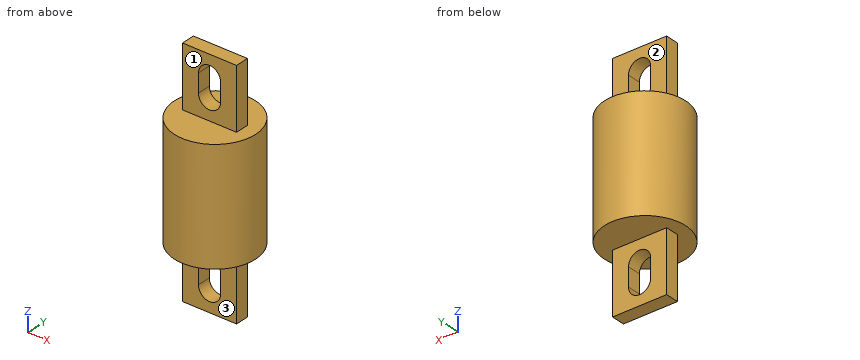
```python
from build123d import *

# Parameters (mm, degrees)
SKETCH1_R       = 19.05
FUSE_DEPTH      = 26.67
FUSE_DEPTH_BACK = 26.67
SKETCH2_W       = 25.4
SKETCH2_H       = 28.575
TAB_DEPTH       = 3.175


with BuildPart() as part:
    # Sketch1 → Fuse (new body, two sides)
    with BuildSketch(Plane.XY) as fuse_sk:
        Circle(SKETCH1_R)
    extrude(amount=FUSE_DEPTH)
    extrude(fuse_sk.sketch, amount=-FUSE_DEPTH_BACK)

    # Sketch2 → Tab (add, symmetric)
    with BuildSketch(Plane(origin=(0, 0, 0), x_dir=(1, 0, 0), z_dir=(0, 1, 0))):
        with Locations((0, 40.9575)):
            Rectangle(SKETCH2_W, SKETCH2_H)
        with BuildLine():
            Line((-5.207, 36.6395), (-5.207, 45.2755))
            ThreePointArc((-5.207, 45.2755), (0, 50.4825), (5.207, 45.2755))
            Line((5.207, 45.2755), (5.207, 36.6395))
            ThreePointArc((5.207, 36.6395), (0, 31.4325), (-5.207, 36.6395))
        make_face(mode=Mode.SUBTRACT)
    tab = extrude(amount=TAB_DEPTH, both=True)

    # Tab Mirror: Tab across plane
    add(tab.mirror(Plane.XY))


solid = part.part
```
Work out the finished part from the listing and answer in its coordinate system (mm). Face numbers are marked on the shaded views. A direction names the side the tool comes from. Give positions to 0.01 mm unless a question says otherwise; leave off trailing zeros. Order: outer loops, then holes, each group sorted by start corner. A loop starts at its lowest first (then second) coordinate and runs counter-clockwise, first axis right, second up. Notation, with made-up numbers: (32, 36.5) - (52, 36.5) arc R19 ccw to (52, 64.5) - close; hole circle Ø2 at (24, -25). An arc over 180 degrees is marked (long way). One line per item, written item: value. Start each with the question number.
1. Section D-D, the plane x = 10 is taken. Write down the section's boundary in (y, z) (3 decimals), then the cut area to 3 significant figures.
2. Each of these flat-tipped pins is pushed along its axis until it touches: pin 1 Ø3 at (y, z) = (-1.5, 41) entering from +X; pin 2 Ø4 at (x, y) = (-2, 13.5) entering from +Z; pin 3 Ø12 at (y, z) = (9.5, -26.5) entering from +X; pin 4 Ø19 at (x, y) = (2, 4.5) entering from +Z (3 decimals). Where does it stop, or does it pass through?
3. Which of the six approach directions +Z, -Z, +X, -X, +Y, -Y give full straight-line access (tool end or side, diameter ignored) to the marked faces 1, 2 and 3?
4. Consider line 1 (Z direction, x = 4, y = 11.5); line 2 (Y direction, x = -6, z = 45.5) (3 decimals); line 3 (Y direction, x = 11.5, z = 12.5). Determine where each line is inside the solid, lowest interval first.
5. Section B-B, the plane z = 42 is taken. Write down the section's boundary in (x, y) (3 decimals), then the cut area to 3 significant figures.
6. Section A-A, the plane y = 0 is taken. Count the separate pieces of the cut face and the enclosed holes in it, then the cut area to 3 significant figures.
Filled sheet:
1. outline: (-16.214, -26.67) - (-3.175, -26.67) - (-3.175, -55.245) - (3.175, -55.245) - (3.175, -26.67) - (16.214, -26.67) - (16.214, 26.67) - (3.175, 26.67) - (3.175, 55.245) - (-3.175, 55.245) - (-3.175, 26.67) - (-16.214, 26.67) - close
1. area: 2,090 mm²
2. pin 1: x = 12.7
2. pin 2: z = 26.67
2. pin 3: x = 18.73
2. pin 4: z = 55.245
3. face 1: +Z, +X, -X, -Y
3. face 2: +Z, +X, -X, +Y
3. face 3: -Z, +X, -X, -Y
4. line 1: -26.67 to 26.67
4. line 2: -3.175 to 3.175
4. line 3: -15.19 to 15.19
5. outline: (-12.7, -3.175) - (-5.207, -3.175) - (-5.207, 3.175) - (-12.7, 3.175) - close; (5.207, -3.175) - (12.7, -3.175) - (12.7, 3.175) - (5.207, 3.175) - close
5. area: 95.2 mm²
6. separate pieces: 1
6. enclosed holes: 2
6. area: 3,130 mm²
